Input: part model. Units: mm. Frame: model coordinates. Face numbers are marked on the shaded views. A direction names the side the tool comes from. Give positions to 0.01 mm unless a question says otherwise; leave off trailing zeros. Loops run counter-clockwise (first coordinate to the right, second up) from the corner with the lowest first, then second, coordinate; pieces in that order, holes last. Notation, with made-up numbers: M -21.5,54 L -15.5,54 A17 ccw -15.5,79 Z; hole C -19,67 d10. An arc over 180 degrees is marked long. Answer as a JSON object with one key per item and string values. Group by question number.
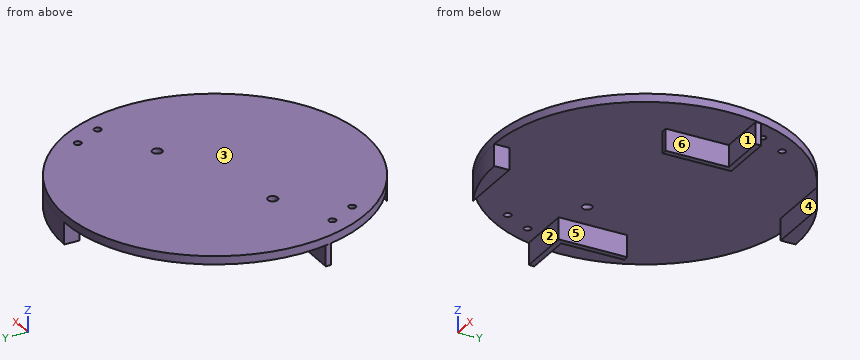
```python
from build123d import *

# Parameters (mm, degrees)
SKETCH_R      = 55
PAD_DEPTH     = 3
SKETCH003_R   = 1.3
SKETCH003_R_2 = 1.8
POCKET_DEPTH  = 5
PAD001_DEPTH  = 11
PAD002_DEPTH  = 11


with BuildPart() as part:
    # Sketch → Pad (new body)
    with BuildSketch(Plane.XY):
        Circle(SKETCH_R)
    extrude(amount=PAD_DEPTH)

    # Sketch003 → Pocket (cut)
    with BuildSketch(Plane.XY.offset(3)):
        with Locations((-45, -18)):
            Circle(SKETCH003_R)
        with Locations((45, 18)):
            Circle(SKETCH003_R)
        with Locations((-40, -28)):
            Circle(SKETCH003_R)
        with Locations((40, 28)):
            Circle(SKETCH003_R)
        with Locations((-23.022469, -8.379494)):
            Circle(SKETCH003_R_2)
        with Locations((23.022469, 8.379494)):
            Circle(SKETCH003_R_2)
    extrude(amount=-POCKET_DEPTH, mode=Mode.SUBTRACT)

    # Sketch001 (on Face3 of Pad) → Pad001 (join)
    with BuildSketch(Plane.XY.offset(3)):
        Polygon((33.500008, 0), (33.500008, 13), (53.345406, 13), (53.345406, 11), (35.5, 11), (35.5, -0.005684), (35.5, -12), (33.500008, -12), align=None)
        Polygon((-33.5, 0), (-33.5, -13), (-53.293575, -13), (-53.293575, -11), (-35.5, -11), (-35.5, 0.001212), (-35.5, 12), (-33.5, 12), align=None)
    extrude(amount=-PAD001_DEPTH)

    # Sketch002 → Pad002 (join)
    with BuildSketch(Plane.XY.offset(3)):
        with BuildLine():
            ThreePointArc((-23.973944, -49.5), (-12.298374, -53.607369), (0, -55))
            Line((0, -49.5), (0, -55))
            Line((-23.973944, -49.5), (0, -49.5))
        make_face()
        with BuildLine():
            ThreePointArc((23.973944, 49.5), (12.298374, 53.607369), (0, 55))
            Line((0, 49.5), (0, 55))
            Line((23.973944, 49.5), (0, 49.5))
        make_face()
    extrude(amount=-PAD002_DEPTH)


solid = part.part
```
1. Reachability of the marked faces 1, 2 and 3 from +Z, -Z, +X, -X, +Y, -Y: full face, straight path, thin tool, end or side. Return the list, or none.
2. Section B-B (x = 40). Output: boundary loops of the cut face in (y, z).
3. Material intervals for L1, parallel to X at y = 0, z = -1.5; L2, parallel to Z at x = -24, y = -28; L3, parallel to Y at x = -50, z = -0.75, sorted ascending.
4. Section A-A (z = -1.25). Output: boundary loops of the cut face in (x, y).
5. Section C-C (y = -18). Output: boundary loops of the cut face in (x, z), then the cut area to 3 significant figures.
6. First-contact query: P1, Ø4, axis at y = -4.5, z = -4, coming from the +X side; P2, Ø3, axis at x = 23.02, y = 8.38, coming from the +Z side (3 decimals); P3, Ø5, axis at y = -5, z = 0, coming from the +X side; P4, Ø1, axis at x = -35, z = -5.5, coming from the +Y side. Flat tips, straight axial feed; report the tip coordinate or a pass-through.
7. Section D-D (y = 0). Output: boundary loops of the cut face in (x, z), then the cut area to 3 significant figures.
8. Mould query, pull axis X, two halves, no side actions, for the marked faces 4, 5 and 6. Classes: pulls with the +X half, pulls with the -X half, needs draft (parallel to the pull), parting line crosses it, or undercut.
Geometry results:
{
 "1": {"face 1": "-Z, +X, -Y", "face 2": "-Z, +X, -X, -Y", "face 3": "+Z, +X, -X, +Y, -Y"},
 "2": {"outline": "M -37.75,0 L 11,0 L 11,-8 L 13,-8 L 13,0 L 26.7,0 L 26.7,3 L -37.75,3 Z; M 29.3,0 L 37.75,0 L 37.75,3 L 29.3,3 Z"},
 "3": {"L1": "-35.5 to -33.5, 33.5 to 35.5", "L2": "0 to 3", "L3": "-13 to -11"},
 "4": {"outline": "M -53.29,-13 L -33.5,-13 L -33.5,12 L -35.5,12 L -35.5,-11 L -53.29,-11 Z; M -23.97,-49.5 A55 ccw 0,-55 L 0,-49.5 Z; M 0,49.5 L 23.97,49.5 A55 ccw 0,55 Z; M 33.5,-12 L 35.5,-12 L 35.5,11 L 53.35,11 L 53.35,13 L 33.5,13 Z"},
 "5": {"outline": "M -51.97,0 L -46.3,0 L -46.3,3 L -51.97,3 Z; M -43.7,0 L 51.97,0 L 51.97,3 L -43.7,3 Z", "area": "304 mm2"},
 "6": {"P1": "x = 35.5", "P2": "through", "P3": "x = 54.94", "P4": "y = 12"},
 "7": {"outline": "M -55,0 L -35.5,0 L -35.5,-8 L -33.5,-8 L -33.5,0 L 33.5,0 L 33.5,-8 L 35.5,-8 L 35.5,0 L 55,0 L 55,3 L -55,3 Z", "area": "362 mm2"},
 "8": {"face 4": "needs draft", "face 5": "undercut", "face 6": "pulls with the +X half"}
}
